from build123d import *

# Parameters (mm, degrees)
CROQUIS1_R              = 1.7
SALIENTE_EXTRUIR1_DEPTH = 5
SALIENTE_EXTRUIR2_DEPTH = 10
CROQUIS3_R              = 2.95
CORTAR_EXTRUIR1_DEPTH   = 3


with BuildPart() as part:
    # Croquis1 → Saliente-Extruir1 (new body)
    with BuildSketch(Plane(origin=(0, 0, 0), x_dir=(1, 0, 0), z_dir=(0, 1, 0))):
        with BuildLine():
            Line((-29.045481576, -3), (-28.039971469, -3))
            ThreePointArc((-28.039971469, -3), (-28.159964448, -1.502132578), (-28.2, 0))
            Line((-28.2, 0), (-21, 0))
            ThreePointArc((-21, 0), (-20.697569753, 3.551141553), (-19.798989873, 7))
            Line((-19.798989873, 7), (-27.317393726, 7))
            ThreePointArc((-27.317393726, 7), (0, 28.2), (27.317393726, 7))
            Line((27.317393726, 7), (19.798989873, 7))
            ThreePointArc((19.798989873, 7), (20.697569753, 3.551141553), (21, 0))
            Line((21, 0), (28.2, 0))
            ThreePointArc((28.2, 0), (28.159964448, -1.502132578), (28.039971469, -3))
            Line((28.039971469, -3), (29.045481576, -3))
            ThreePointArc((29.045481576, -3), (0, 29.2), (-29.045481576, -3))
        make_face()
        with Locations((-25, 3.5)):
            Circle(CROQUIS1_R, mode=Mode.SUBTRACT)
        with Locations((25, 3.5)):
            Circle(CROQUIS1_R, mode=Mode.SUBTRACT)
    extrude(amount=SALIENTE_EXTRUIR1_DEPTH)

    # Croquis2 → Saliente-Extruir2 (add)
    with BuildSketch(Plane(origin=(0, 5, 0), x_dir=(1, 0, 0), z_dir=(0, 1, 0))):
        with BuildLine():
            Line((28.039971469, -3), (29.045481576, -3))
            ThreePointArc((29.045481576, -3), (21.848911842, 19.371759118), (0.5, 29.195718864))
            Line((0.5, 29.195718864), (0.5, 28.195567027))
            ThreePointArc((0.5, 28.195567027), (21.140561568, 18.663243464), (28.039971469, -3))
        make_face()
        with BuildLine():
            Line((-29.045481576, -3), (-28.039971469, -3))
            ThreePointArc((-28.039971469, -3), (-21.140561568, 18.663243464), (-0.5, 28.195567027))
            Line((-0.5, 28.195567027), (-0.5, 29.195718864))
            ThreePointArc((-0.5, 29.195718864), (-21.848911842, 19.371759118), (-29.045481576, -3))
        make_face()
    extrude(amount=SALIENTE_EXTRUIR2_DEPTH)

    # Croquis3 → Cortar-Extruir1 (cut)
    with BuildSketch(Plane(origin=(0, 5, 0), x_dir=(1, 0, 0), z_dir=(0, 1, 0))):
        with Locations((-25, 3.5)):
            Circle(CROQUIS3_R)
        with Locations((25, 3.5)):
            Circle(CROQUIS3_R)
    extrude(amount=-CORTAR_EXTRUIR1_DEPTH, mode=Mode.SUBTRACT)


solid = part.part
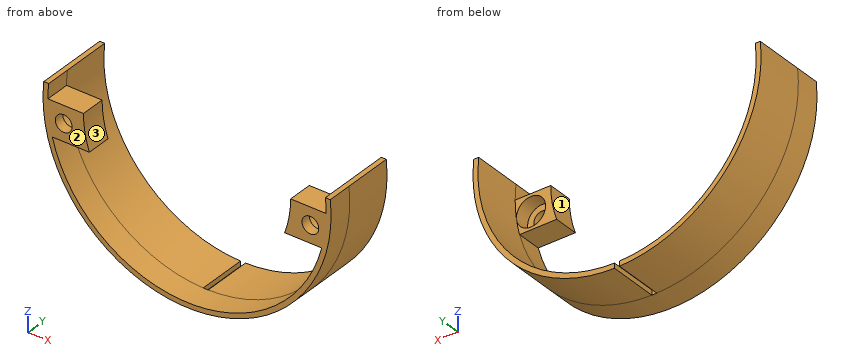
Read the model definition and answer for the solid it produces. Units are mm, in the model's axes. Face numbers are marked on the shaded views. Give positions to 0.01 mm unless a question says otherwise; leave off trailing zeros. Loops run counter-clockwise (first coordinate to the right, second up) from the corner with the lowest first, then second, coordinate; pieces in that order, holes last. Notation, with made-up numbers: (-3, 40) - (44, 40) arc R22 ccw to (44, 65) - close; hole circle Ø9 at (87.25, -30.75). An arc over 180 degrees is marked (long way). Answer as CSV lines item,"result". Start each with the question number.
1) Straight lines are drawn through the part: L1, parallel to X at y = 1.05, z = -3.5; L2, parallel to X at y = 3.75, z = -3.5; L3, parallel to Z at x = 25, y = 0.65. For each, find the intervals that lie inside material, in ascending order. Write a range as from..to.
2) Each of these flat-tipped pins is pushed along its axis until it touches: pin 1 Ø5.5 at (x, z) = (23.5, -4.5) entering from +Y; pin 2 Ø8 at (x, y) = (-1.5, 12.5) entering from -Z; pin 3 Ø5.5 at (x, y) = (23, 3.5) entering from +Z; pin 4 Ø2 at (x, z) = (25, -3.5) entering from +Y (3 decimals). Where does it stop, or does it pass through?
3) Find section C-C (x = 25). Write down the section's boundary in (y, z), then the cut area to 3 significant figures.
4) Determine the mould class of the marked faces 1, 2 and 3 for opening direction X: released by +X, released by -X, zero draft, split by the parting line, or undercut.
5) Find section D-D (z = -3.5). State how many separate pieces and enclosed holes the cut face has, then the cut area to 3 significant figures.
6) Find section B-B (y = 7). Write down the section's boundary in (x, z).
7) Find section A-A (z = -12.5). Write down the section's boundary in (x, y), then the cut area to 3 significant figures.
Findings below:
1,L1,"-28.99..-26.7, -23.3..-20.71, 20.71..23.3, 26.7..28.99"
1,L2,"-28.99..-27.95, -22.05..-20.71, 20.71..22.05, 27.95..28.99"
1,L3,"-15.09..-13.05, -7..-5.2, -1.8..0"
2,pin 1,"y = 5"
2,pin 2,"z = -29.2"
2,pin 3,"z = 0"
2,pin 4,"through"
3,outline,"(0, -15.09) - (15, -15.09) - (15, -13.05) - (0, -13.05) - close; (0, -7) - (5, -7) - (5, -6.45) - (2, -6.45) - (2, -5.2) - (0, -5.2) - close; (0, -1.8) - (2, -1.8) - (2, -0.55) - (5, -0.55) - (5, 0) - (0, 0) - close"
3,area,"41.1 mm^2"
4,face 1,"undercut"
4,face 2,"zero draft"
4,face 3,"undercut"
5,separate pieces,"4"
5,enclosed holes,"0"
5,area,"54.0 mm^2"
6,outline,"(-29.05, 3) arc R29.2 ccw to (-0.5, -29.2) - (-0.5, -28.2) arc R28.2 cw to (-28.04, 3) - close; (0.5, -29.2) arc R29.2 ccw to (29.05, 3) - (28.04, 3) arc R28.2 cw to (0.5, -28.2) - close"
7,outline,"(-26.39, 0) - (-25.28, 0) - (-25.28, 15) - (-26.39, 15) - close; (25.28, 0) - (26.39, 0) - (26.39, 15) - (25.28, 15) - close"
7,area,"33.3 mm^2"
